Design review of the part built by this model. Coordinates are the model's own, in mm. Face numbers are marked on the shaded views. A direction names the side the tool comes from. Give positions to 0.01 mm unless a question says otherwise; leave off trailing zeros. Loops run counter-clockwise (first coordinate to the right, second up) from the corner with the lowest first, then second, coordinate; pieces in that order, holes last. Notation, with made-up numbers: M 0,3.25 L 17,3.25 A26 cw 17,17.25 Z; hole C 24,-2.5 d8. An arc over 180 degrees is marked long. Use CSV: the item, a comma, the result in double quotes.
from build123d import *

# Parameters (mm, degrees)
SKETCH1_W           = 17
SKETCH1_H           = 32
SKETCH1_R           = 2.5
BOSS_EXTRUDE1_DEPTH = 5
SKETCH2_R           = 6
SKETCH2_R_2         = 4
BOSS_EXTRUDE2_DEPTH = 15
FILLET1_R           = 1


with BuildPart() as part:
    # Sketch1 → Boss-Extrude1 (new body)
    with BuildSketch(Plane(origin=(0, 0, 0), x_dir=(1, 0, 0), z_dir=(0, 1, 0))):
        Rectangle(SKETCH1_W, SKETCH1_H)
        with Locations((0, 11.5)):
            Circle(SKETCH1_R, mode=Mode.SUBTRACT)
        with Locations((0, -11.5)):
            Circle(SKETCH1_R, mode=Mode.SUBTRACT)
    extrude(amount=BOSS_EXTRUDE1_DEPTH)

    # Sketch2 → Boss-Extrude2 (add)
    with BuildSketch(Plane(origin=(0, 5, 0), x_dir=(1, 0, 0), z_dir=(0, 1, 0))):
        Circle(SKETCH2_R)
        Circle(SKETCH2_R_2, mode=Mode.SUBTRACT)
    extrude(amount=BOSS_EXTRUDE2_DEPTH)

    # Fillet1
    fillet1_edges = [part.edges().sort_by_distance(p)[0] for p in [
        (-8.5, 5, 0),
        (0, 5, 16),
        (8.5, 5, 0),
        (0, 5, -16),
    ]]
    fillet(fillet1_edges, radius=FILLET1_R)


solid = part.part
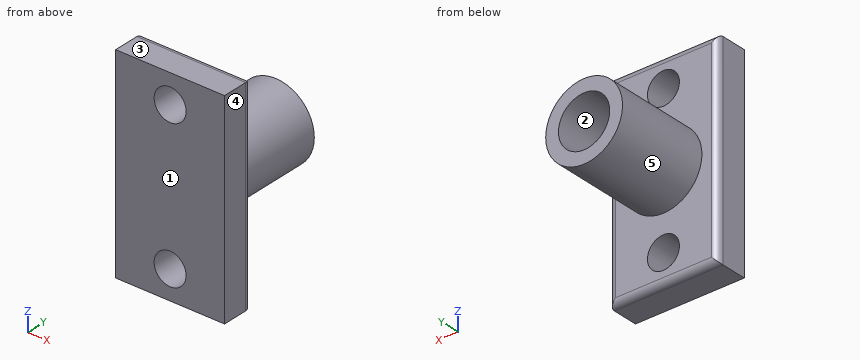
(1) We need section D-D on z = 0. State the section outline as (x, y) points, then the cut area to 3 significant figures.
A:
outline,"M -8.5,0 L 8.5,0 L 8.5,4 A1 ccw 7.5,5 L 6,5 L 6,20 L 4,20 L 4,5 L -4,5 L -4,20 L -6,20 L -6,5 L -7.5,5 A1 ccw -8.5,4 Z"
area,"145 mm²"
(2) We need section C-C on y = 12. State the section outline as (x, z) points.
A:
outline,"C 0,0 d12; hole C 0,0 d8"
(3) We need section A-A on z = 11.5. State the section outline as (x, y) points.
A:
outline,"M -8.5,0 L -2.5,0 L -2.5,5 L -7.5,5 A1 ccw -8.5,4 Z; M 2.5,0 L 8.5,0 L 8.5,4 A1 ccw 7.5,5 L 2.5,5 Z"
(4) Wall thickness on line 1 along Z through (x, y) = (0, 3.55); line 2 along Z through (x, y) = (0, 10.25); line 3 along Z through (x, y) = (1, 4): over which ranges is each line inside the solid? List them lowest first. Write a range as [from, to].
A:
line 1,"[-16, -14], [-9, 9], [14, 16]"
line 2,"[-6, -4], [4, 6]"
line 3,"[-16, -13.79], [-9.21, 9.21], [13.79, 16]"
(5) The part is to be moulded in two halves that separate along Z. For the marked faces 1, 2 and 3, say which applies: released by +Z, released by -Z, zero draft, split by the parting line, or undercut.
A:
face 1,"zero draft"
face 2,"undercut"
face 3,"released by +Z"
(6) We need section B-B on x = 0. State the section outline as (y, z) points, then the cut area to 3 significant figures.
A:
outline,"M 0,-16 L 4,-16 A1 ccw 5,-15 L 5,-14 L 0,-14 Z; M 0,-9 L 5,-9 L 5,-6 L 20,-6 L 20,-4 L 5,-4 L 5,4 L 20,4 L 20,6 L 5,6 L 5,9 L 0,9 Z; M 0,14 L 5,14 L 5,15 A1 ccw 4,16 L 0,16 Z"
area,"170 mm²"
(7) Clearance check with flat-ended pins moving along their axes: P1, Ø2, axis at x = -5, z = -6, coming from the +Y side; P2, Ø2, axis at x = 5, y = 13, coming from the +Z side; P3, Ø4, axis at x = -5, y = 13.5, coming from the +Z side. State where each tip first meets the part, or that it passes through.
A:
P1,"y = 5"
P2,"z = 4.47"
P3,"z = 5.2"
(8) Machinability: for the marked faces 4 and 5, which of the approach directions +Z, -Z, +X, -X, +Y, -Y give a long, thin tool a straight path to every point of the face, cutting with its end or side? Answer none if there is none.
A:
face 4,"+Z, -Z, +X, +Y, -Y"
face 5,"+Y"
